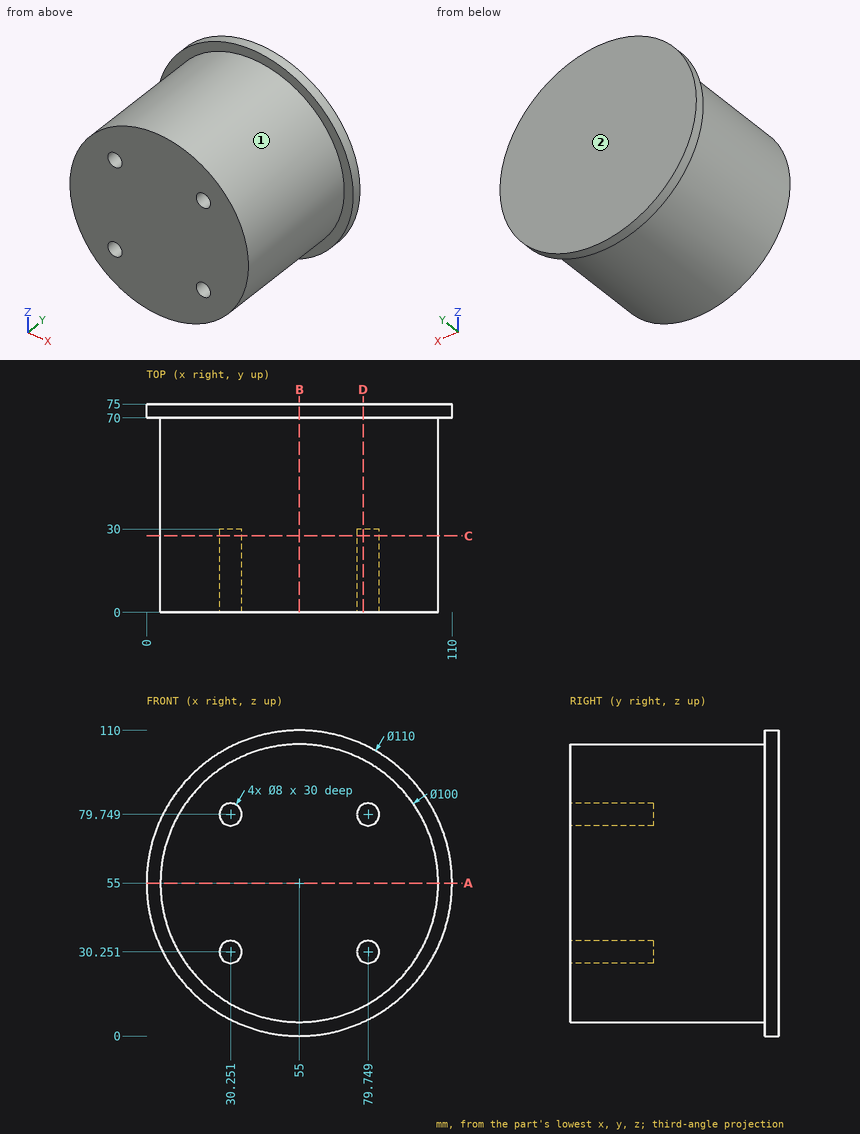
Here's the drawing with two shaded views (mm, measured from the low corner). I have some questions. A direction names the side the tool comes from. Give positions to 0.01 mm unless a question says otherwise; leave off trailing zeros. Write each loop counter-clockwise with the first axis right and the second up, starting at its lowest first coordinate (ties: lowest second). Pieces come first, ordered by that corner, then holes. Notation, with made-up numbers: (-11, 43) -> (16, 43) arc R17 ccw to (16, 47) -> close; hole circle Ø6 at (52, 9). An arc over 180 degrees is marked (long way). Use one line per item in the form item = value.
1) Suppose I cut it at D-D (x = 78). Please give me the cut outline in (y, z).
Verdict:
outline = (0, 10.6) -> (70, 10.6) -> (70, 5.04) -> (75, 5.04) -> (75, 104.96) -> (70, 104.96) -> (70, 99.4) -> (0, 99.4) -> (0, 83.35) -> (30, 83.35) -> (30, 76.15) -> (0, 76.15) -> (0, 33.85) -> (30, 33.85) -> (30, 26.65) -> (0, 26.65) -> close
2) If I drill on L1, parallel to X at y = 10, z = 30; L2, parallel to X at y = 18, z = 28 (1 decimal); L3, parallel to X at y = 50.5, z = 54, over which ranges is the centre line in solid material (lowest first)? Write a range as [from, to].
Verdict:
L1 = [11.7, 26.26], [34.24, 75.76], [83.74, 98.3]
L2 = [12.9, 26.9], [33.6, 76.4], [83.1, 97.1]
L3 = [5.01, 104.99]
3) Suppose I cut it at A-A (z = 55). Please give me the cut outline in (x, y).
Verdict:
outline = (0, 70) -> (5, 70) -> (5, 0) -> (105, 0) -> (105, 70) -> (110, 70) -> (110, 75) -> (0, 75) -> close
4) I'm going to push flat-ended pins straight in: pin 1 (5 mm diameter, centred on y = 44.5, z = 57, fed in from -X); pin 2 (5 mm diameter, centred on y = 39, z = 72.5, fed in from -X); pin 3 (3 mm diameter, centred on y = 42.5, z = 62, fed in from -X). Where does each tip first touch, or does it pass through?
Verdict:
pin_1 = 5
pin_2 = 7.3
pin_3 = 5.3
5) Suppose I cut it at B-B (x = 55). Please give me the cut outline in (y, z), and give its area (3 significant figures).
Verdict:
outline = (0, 5) -> (70, 5) -> (70, 0) -> (75, 0) -> (75, 110) -> (70, 110) -> (70, 105) -> (0, 105) -> close
area = 7,550 mm2
6) On a 3-axis mill with a long thin cutter (end or side, diameter ignored), from which of +Z, -Z, +X, -X, +Y, -Y can I reach the whole of each face in a straight line? I mean the marked faces 1 and 2. Say none if no direction works.
Verdict:
face_1 = -Y
face_2 = +Z, -Z, +X, -X, +Y
7) Suppose I cut it at C-C (y = 27.5). Please give me the cut outline in (x, z), and give its area (3 significant figures).
Verdict:
outline = circle Ø100 at (55, 55); hole circle Ø8 at (30.25, 30.25); hole circle Ø8 at (30.25, 79.75); hole circle Ø8 at (79.75, 30.25); hole circle Ø8 at (79.75, 79.75)
area = 7,650 mm2
